Geometry: final body of the model. Coordinates: model frame, mm. A direction names the side the tool comes from. Give positions to 0.01 mm unless a question says otherwise; leave off trailing zeros. Order: outer loops, then holes, each group sorted by start corner. A loop starts at its lowest first (then second) coordinate and runs counter-clockwise, first axis right, second up. Notation, with made-up numbers: (-39, 22) -> (0, 22) arc R24 ccw to (0, 54) -> close; hole circle Ø3 at (39.5, 11.25). An arc over 180 degrees is marked (long way). One line per question, with ' | ' between items.
from build123d import *

# Parameters (mm, degrees)
F1_DEPTH = 5.08
F2_R     = 1.905
F3_DEPTH = 5.081


with BuildPart() as f1:
    # F0 (on Top) → F1 (new body)
    with BuildSketch(Plane.XY):
        with BuildLine():
            Line((0, 0), (12.7, 0))
            ThreePointArc((12.7, 0), (12.5987771426, 1.6002545145), (12.2967221242, 3.175))
            Line((12.2967221242, 3.175), (6.1483610621, 3.175))
            Line((6.1483610621, 3.175), (0, 3.175))
            Line((0, 3.175), (0, 0))
        make_face()
        with BuildLine():
            ThreePointArc((12.2967221242, -3.175), (12.5987771426, -1.6002545145), (12.7, 0))
            Line((12.7, 0), (0, 0))
            Line((0, 0), (0, -3.175))
            Line((0, -3.175), (6.1483610621, -3.175))
            Line((6.1483610621, -3.175), (12.2967221242, -3.175))
        make_face()
        with BuildLine():
            Line((6.1483610621, 3.175), (12.2967221242, 3.175))
            ThreePointArc((12.2967221242, 3.175), (11.1125, 6.1483610621), (9.2225415932, 8.73125))
            Line((9.2225415932, 8.73125), (6.1483610621, 3.175))
        make_face()
        with BuildLine():
            Line((-12.7, 0), (0, 0))
            Line((0, 0), (0, 3.175))
            Line((0, 3.175), (0, 6.35))
            Line((0, 6.35), (0, 12.7))
            ThreePointArc((0, 12.7), (-8.9802561211, 8.9802561211), (-12.7, 0))
        make_face()
        with BuildLine():
            Line((0, -3.175), (0, 0))
            Line((0, 0), (-12.7, 0))
            ThreePointArc((-12.7, 0), (-8.9802561211, -8.9802561211), (0, -12.7))
            Line((0, -12.7), (0, -6.35))
            Line((0, -6.35), (0, -3.175))
        make_face()
    extrude(amount=F1_DEPTH)

    # F2 (on face) → F3 (cut, through all)
    with BuildSketch(Plane.XY.offset(5.08)):
        with Locations((-3.81, 0)):
            Circle(F2_R)
    extrude(amount=-F3_DEPTH, mode=Mode.SUBTRACT)


solid = f1.part
1) Set-up query: faces 4 (the flat face through (0, 0, 5.08)), 5 (the flat face through (6, -3.175, 3)), 6 (the flat face through (3, 3.175, 3)). Return all of +Z, -Z, +X, -X, +Y, -Y with unobstructed straight access to the full face (end or side cutting, diameter ignored); none if empty.
Check result:
face 4: +Z, +X, -X, +Y, -Y | face 5: +Z, -Z, +X, -Y | face 6: +Z, -Z, +Y
2) Material intervals for probe 1 along X at (y, z) = (0.5, 2.2); probe 2 along Y at (x, z) = (2.75, 1.3) (3 decimals); probe 3 along Y at (x, z) = (-2.75, 3.55), sorted ascending. Write a range as from..to.
Check result:
probe 1: x = -12.69..-5.65, -1.97..12.69 | probe 2: y = -3.175..3.175 | probe 3: y = -12.4..-1.58, 1.58..12.4
3) Section B-B on z = 4.4. Return loops of the section in (x, y) (3 decimals), plus the area to 3 significant figures.
Check result:
outline: (0, -12.7) -> (0, -3.175) -> (12.297, -3.175) arc R12.7 ccw to (9.223, 8.731) -> (6.148, 3.175) -> (0, 3.175) -> (0, 12.7) arc R12.7 ccw to start; hole circle Ø3.81 at (-3.81, 0) | area: 341 mm^2
4) Section C-C on y = 5. Return loops of the section in (x, z), plus the area to 3 significant figures.
Check result:
outline: (-11.67, 0) -> (0, 0) -> (0, 5.08) -> (-11.67, 5.08) -> close; (7.16, 0) -> (11.67, 0) -> (11.67, 5.08) -> (7.16, 5.08) -> close | area: 82.2 mm^2
5) Pull-direction query (X, two-part tool) for faces 1 (the flat face through (0, 8, 3)), 2 (the flat face through (0, 0, 0)), 3 (the flat face through (0, -8, 3)); classes: +X half, -X half, draft (parallel to the pull), parting line (faces both ways), or undercut.
Check result:
face 1: undercut | face 2: draft | face 3: +X half
6) Section A-A on x = -3.81. Return loops of the section in (y, z) (3 decimals), plus the area to 3 significant figures.
Check result:
outline: (-12.115, 0) -> (-1.905, 0) -> (-1.905, 5.08) -> (-12.115, 5.08) -> close; (1.905, 0) -> (12.115, 0) -> (12.115, 5.08) -> (1.905, 5.08) -> close | area: 104 mm^2
7) Contact query for flat-ended pins moving along their axis: pin 1 Ø1.5 at (y, z) = (8, 1.5) entering from +X; pin 2 Ø1.5 at (x, z) = (3, 3) entering from -Y (3 decimals). Output: stop coordinate, or through.
Check result:
pin 1: stops at x = 10.43 | pin 2: stops at y = -3.175
8) Section D-D on x = 4.25. Return loops of the section in (y, z) (3 decimals).
Check result:
outline: (-3.175, 0) -> (3.175, 0) -> (3.175, 5.08) -> (-3.175, 5.08) -> close
